Read the model definition and answer for the solid it produces. Units are mm, in the model's axes. Face numbers are marked on the shaded views. A direction names the side the tool comes from. Coordinates: 2 decimals unless noted, no trailing zeros. Loops run counter-clockwise (first coordinate to the right, second up) from the corner with the lowest first, then second, coordinate; pieces in that order, holes last. Notation, with made-up numbers: (38.5, 66.25) -> (74.5, 66.25) arc R11 ccw to (74.5, 77.25) -> close; hole circle Ø1 at (64, 11). An arc over 180 degrees is marked (long way). Answer as a JSON object with one key per item and string values. Group by question number.
Q1. The part is cut by section A-A on x = -1.5. Write down the section's boundary in (y, z).
Q2. Straight lines are drawn through the part: line 1 along Z through (x, y) = (-9.5, -22.25); line 2 along X through (y, z) = (-3, -18); line 3 along X through (y, z) = (-20.25, -27). For each, find the intervals that lie inside material, in ascending order. Write a range as [from, to].
Q3. The part is cut by section C-C on z = 19.5. Write down the section's boundary in (x, y).
Q4. Each of these flat-tipped pins is pushed along its axis until it touches: P1, Ø1, axis at y = -22.5, z = -26.5, coming from the -X side; P2, Ø12.5, axis at x = -25.5, y = -18, coming from the -Z side; P3, Ø6, axis at y = -11, z = -22, coming from the -X side. Where does it stop, or does it pass through?
Q5. The part is cut by section B-B on y = -20. Write down the section's boundary in (x, z) (3 decimals), and give its area (3 significant figures).
Q6. For the marked faces 1, 2 and 3, determine the directions among +Z, -Z, +X, -X, +Y, -Y from which every point of the face is accessible in a straight line to the end or side of a thin tool.
Q7. The part is cut by section D-D on x = 26. Write down the section's boundary in (y, z), and give its area (3 significant figures).
Q8. Determine the mould class of the marked faces 4, 5, 6 and 7 for opening direction X: released by +X, released by -X, zero draft, split by the parting line, or undercut.
from build123d import *

# Parameters (mm, degrees)
F1_DEPTH = 25.4


with BuildPart() as f1:
    # F0 (on Front) → F1 (new body)
    with BuildSketch(Plane.XZ):
        Polygon((-44.430528, -31.197766), (-18.49081, -31.197766), (-12.18115, 0), (8.500515, 0), (20.594032, -33.300985), (54.420825, -33.300985), (35.66711, -27.517129), (14.985446, 26.46552), (22.521986, 32.95045), (-17.965006, 32.95045), (-33.56389, -27.517129), align=None)
        Polygon((-9.727393, 25.063373), (3.067197, 25.063373), (7.650744, 13.09954), (10.117609, 6.660604), (-14.109102, 6.660604), align=None, mode=Mode.SUBTRACT)
    extrude(amount=F1_DEPTH)


solid = f1.part
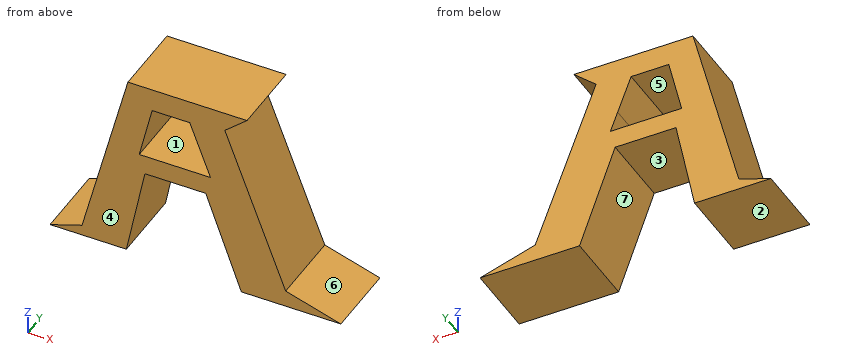
Final values:
{
 "1": {"outline": "(-25.4, 0) -> (0, 0) -> (0, 6.66) -> (-25.4, 6.66) -> close; (-25.4, 25.06) -> (0, 25.06) -> (0, 32.95) -> (-25.4, 32.95) -> close"},
 "2": {"line 1": "z = [0, 6.66], [25.06, 32.95]", "line 2": "x = [-31.11, -15.82], [15.04, 32.02]", "line 3": "x = [-33.43, -17.64], [18.31, 35.47]"},
 "3": {"outline": "(-21.43, -25.4) -> (-11.05, -25.4) -> (-11.05, 0) -> (-21.43, 0) -> close; (5.2, -25.4) -> (17.65, -25.4) -> (17.65, 0) -> (5.2, 0) -> close"},
 "4": {"P1": "stops at x = -33.43", "P2": "stops at z = -31.2", "P3": "stops at x = -32.91"},
 "5": {"outline": "(-44.431, -31.198) -> (-18.491, -31.198) -> (-12.181, 0) -> (8.501, 0) -> (20.594, -33.301) -> (54.421, -33.301) -> (35.667, -27.517) -> (14.985, 26.466) -> (22.522, 32.95) -> (-17.965, 32.95) -> (-33.564, -27.517) -> close; hole (-14.109, 6.661) -> (10.118, 6.661) -> (3.067, 25.063) -> (-9.727, 25.063) -> close", "area": "2,150 mm2"},
 "6": {"face 1": "+Y, -Y", "face 2": "-Z, -X, +Y, -Y", "face 3": "-Z, +Y, -Y"},
 "7": {"outline": "(-25.4, -33.3) -> (0, -33.3) -> (0, -2.28) -> (-25.4, -2.28) -> close", "area": "788 mm2"},
 "8": {"face 4": "zero draft", "face 5": "undercut", "face 6": "released by +X", "face 7": "undercut"}
}
